Part model, mm, in its own coordinate system. A direction names the side the tool comes from. Round coordinates to 2 decimals unless told otherwise and drop trailing zeros. Order: outer loops, then holes, each group sorted by start corner. A loop starts at its lowest first (then second) coordinate and runs counter-clockwise, first axis right, second up. Notation, with made-up numbers: M 77,2 L 117,2 A13 ccw 117,20 Z; hole C -32,-18.75 d10. An arc over 180 degrees is marked long. One line per question, with ' | ' between items.
from build123d import *

# Parameters (mm, degrees)
SKETCH4_W           = 24.633837396
SKETCH4_H           = 19.082768461
SKETCH4_W_2         = 5
SKETCH4_H_2         = 5
MAINBRACKET_DEPTH   = 3.5
SKETCH3_R           = 2
BOSS_EXTRUDE2_DEPTH = 13
SKETCH6_R           = 1.5
BOSS_EXTRUDE3_DEPTH = 5


with BuildPart() as part:
    # Sketch4 → MainBracket (new body)
    with BuildSketch(Plane(origin=(0, 0, 0), x_dir=(1, 0, 0), z_dir=(0, 1, 0))):
        Polygon((-25.001052975, 23.597895529), (25.52718448, 23.597895529), (27.52718448, 21.597895529), (27.52718448, 18.397895529), (25.52718448, 16.397895529), (15.338231538, 16.397895529), (15.338231538, -31.590979949), (12.338231538, -34.590979949), (8.051942307, -34.590979949), (5.051942307, -31.590979949), (5.051942307, -25.634971446), (-16.583029139, -4), (-16.583029139, 16.421906692), (-25.001052975, 16.421906692), (-27.001052975, 18.421906692), (-27.001052975, 21.597895529), align=None)
        with Locations((0.008956485, 13.000441896)):
            Rectangle(SKETCH4_W, SKETCH4_H, mode=Mode.SUBTRACT)
        Polygon((-12.927683275, -4), (8.707288171, -25.634971446), (8.707288171, -29.300035445), (12.325875183, -29.300035445), (12.325875183, -4), align=None, mode=Mode.SUBTRACT)
        Rectangle(SKETCH4_W_2, SKETCH4_H_2, mode=Mode.SUBTRACT)
    extrude(amount=MAINBRACKET_DEPTH)

    # Sketch3 → Boss-Extrude2 (add)
    with BuildSketch(Plane(origin=(0, 0, 0), x_dir=(1, 0, 0), z_dir=(0, 1, 0))):
        with Locations(Location((-24.011269627, 19.663273311, 0), (0, 0, 270))):
            Circle(SKETCH3_R)
        with Locations(Location((24.107482847, 18.27469294, 0), (0, 0, 270))):
            Circle(SKETCH3_R)
        with Locations(Location((8.917908931, -32.088026328, 0), (0, 0, 270))):
            Circle(SKETCH3_R)
    extrude(amount=-BOSS_EXTRUDE2_DEPTH)

    # Sketch6 → Boss-Extrude3 (add)
    with BuildSketch(Plane.XZ.offset(13)):
        with Locations(Location((-24.011269627, -19.663273311, 0), (0, 0, 270))):
            Circle(SKETCH6_R)
        with Locations(Location((8.917908931, 32.088026328, 0), (0, 0, 270))):
            Circle(SKETCH6_R)
        with Locations(Location((24.107482847, -18.27469294, 0), (0, 0, 270))):
            Circle(SKETCH6_R)
    extrude(amount=BOSS_EXTRUDE3_DEPTH)


solid = part.part
1) Two-plate mould, pull along Z, no slides. Class faces 1 (the face through (0, 2, -22.542)), 2 (the face through (-5.614, 1.726, 14.969)), 3 (the face through (0, 3.5, -3)): released by +Z, released by -Z, zero draft, split by the parting line, or undercut.
The answers:
face 1: undercut | face 2: released by +Z | face 3: zero draft
2) Saw through at D-D (y = -11). List the corners of the cut face in (x, z).
The answers:
outline: C -24.01,-19.66 d4; C 8.92,32.09 d4; C 24.11,-18.27 d4
3) Probe line 1 (X direction, y = 0.5, z = 0.5); line 2 (Y direction, x = -14.5, z = 1.5); line 3 (X direction, y = -0.5, z = -19). List the from-to ranges inside material, lowest first. Write a range as [from, to].
The answers:
line 1: x = [-16.58, -2.5], [2.5, 15.34] | line 2: y = [0, 3.5] | line 3: x = [-25.9, -22.12], [22.24, 25.97]
4) Saw through at A-A (z = -1.5). List the corners of the cut face in (x, y).
The answers:
outline: M -16.58,0 L -2.5,0 L -2.5,3.5 L -16.58,3.5 Z; M 2.5,0 L 15.34,0 L 15.34,3.5 L 2.5,3.5 Z
5) Saw through at B-B (x = -7). List the corners of the cut face in (y, z), plus the area to 3 significant figures.
The answers:
outline: M 0,-23.6 L 3.5,-23.6 L 3.5,-22.54 L 0,-22.54 Z; M 0,-3.46 L 3.5,-3.46 L 3.5,4 L 0,4 Z; M 0,9.93 L 3.5,9.93 L 3.5,13.58 L 0,13.58 Z | area: 42.6 mm²
6) Saw through at C-C (y = 1.25). Give the number of separate pieces and of enclosed holes in the cut face, plus the area to 3 significant figures.
The answers:
separate pieces: 1 | enclosed holes: 3 | area: 755 mm²
7) Drop flat-ended pins along their axis: pin 1 (1 mm diameter, centred on y = 1.5, z = 0, fed in from -X); pin 2 (1.8 mm diameter, centred on y = 2, z = 22.5, fed in from -X); pin 3 (4 mm diameter, centred on x = 11, y = -7.5, fed in from -Z). Give the stop position or say it passes through.
The answers:
pin 1: stops at x = -16.58 | pin 2: stops at x = 1.02 | pin 3: stops at z = 30.09
8) Which spindle directions (+Z, -Z, +X, -X, +Y, -Y) get a long thin tool onto all of the face, cutting with end or side? Do faces 4 (the face through (-24.92, -15.46, -18.47)), 5 (the face through (-21, 2, -16.422)), 6 (the face through (12.326, 2, 17)), 7 (the face through (-27.001, 2, -20)). Say none if no direction does.
The answers:
face 4: -Y | face 5: +Z, -X, +Y, -Y | face 6: +Y, -Y | face 7: +Z, -Z, -X, +Y, -Y
